Autodesk Inventor part; units mm, degrees
ref_plane "YZ Plane" through (0, 0, 0) normal (1, 0, 0) x (0, 1, 0)
ref_plane "XZ Plane" through (0, 0, 0) normal (0, 1, 0) x (-1, 0, 0)
ref_plane "XY Plane" through (0, 0, 0) normal (0, 0, 1) x (1, 0, 0)
sketch "Sketch2" plane through (0, 0, 0) normal (0, 0, 1) x (1, 0, 0)
  circle A0 centre (0, 0) radius 18.5
  circle A1 centre (38, 0) radius 6.3
  circle A2 centre (0, 0) radius 6.3
  circle A3 centre (38, 0) radius 18.5
  line L0 (-1.1534, 0) -> (34.5511, 0)
  arc A4 (12.005, 14.0759) -> (25.995, 14.0759) centre (19, 22.2775) ccw
  arc A5 (25.995, -14.0759) -> (12.005, -14.0759) centre (19, -22.2775) ccw
  line L1 (1.1428, -18.5) -> (0, -18.5)
  line L2 (1.1428, 18.5) -> (0, 18.5)
  point P0 (38, 18.5)
  point P1 (38, -18.5)
  point P2 (18.5, 0)
  dimension "d0" = 37
  dimension "d19" = 12.6
  dimension "d20" = 37
  dimension "d26" = 38
extrude "Extrusion1" add sketch "Sketch2" along normal blind 4.3
sketch "Sketch3" plane through (0, 0, 4.3) normal (0, 0, 1) x (1, 0, 0)
  circle A0 centre (38, 0) radius 6.3
  line L0 (38, 0) -> (38, 2.8384)
  point P0 (0, 0)
  point P1 (46.7, 0)
  point P2 (18.9, 0)
  dimension "d7" = 27.8
  dimension "d16" = 8.7
hole "Hole1" at (46.7, 0, 4.3) at (18.9, 0, 4.3) direction (0, 0, -1) diameter 2 depth 7
sketch "Sketch4" plane through (0, 0, 0) normal (0, 0, -1) x (-1, 0, 0)
  circle A0 centre (0, 0) radius 6.3
  line L0 (0, 3.334) -> (0, -2.474)
  line L1 (-2.132, 0) -> (2.0257, 0)
  line L2 (-4.2951, 19.0635) -> (4.2951, 19.0635)
  line L3 (4.2951, 19.0635) -> (4.2951, -19.0635)
  line L4 (4.2951, -19.0635) -> (-4.2951, -19.0635)
  line L5 (-4.2951, -19.0635) -> (-4.2951, 19.0635)
  point P0 (4.2951, -4.609)
  point P1 (-4.2951, -4.609)
  point P2 (-4.2951, 4.609)
  point P3 (4.2951, 4.609)
extrude "Extrusion2" cut sketch "Sketch4" against normal blind 2 contours A0 L5 L2 L3 | L3 L4 L5 A0
sketch "Sketch5" plane through (0, 0, 4.3) normal (0, 0, 1) x (1, 0, 0)
  circle A0 centre (38, 0) radius 6.3
  line L0 (38, 0) -> (38, 11.0593)
  line L1 (38, 0) -> (42.2148, 0)
  line L2 (21.1, 6.5) -> (44.1, 6.5)
  line L3 (44.1, 6.5) -> (44.1, -6.5)
  line L4 (44.1, -6.5) -> (21.1, -6.5)
  line L5 (21.1, -6.5) -> (21.1, 6.5)
  circle A1 centre (46.7, 0) radius 1
  point P0 (0, 0)
  point P1 (44.1, -1.5748)
  point P2 (44.1, 1.5748)
  dimension "d21" = 13
  dimension "d22" = 23
  dimension "d23" = 2.6
extrude "Extrusion3" cut sketch "Sketch5" against normal blind 4.3 contours A0 L0 L2 L3 | L3 L4 L5 L2 L0 A0
fillet "Fillet1" radius 1 14 edges at (19, 11.498, 0) (8.3822, 16.4921, 0) (19, -11.498, 0) (8.3822, -16.4921, 0) (56.5, 0, 0) (-18.5, 0, 0) (19, -11.498, 4.3) (56.5, 0, 4.3) (19, 11.498, 4.3) (-18.5, 0, 4.3) (4.2951, 11.3017, 0) (4.2951, -11.3017, 0) (-4.2951, 11.3017, 0) (-4.2951, -11.3017, 0)
sketch "Sketch7" plane through (0, 0, 2) normal (0, 0, -1) x (-1, 0, 0)
  circle A0 centre (0, 0) radius 6.3
  line L0 (0, 0) -> (0, 23.1769)
  line L1 (0, 0) -> (3.1147, 0)
  point P0 (0, 13.1)
  point P1 (0, -13.1)
  dimension "d28" = 26.2
hole "Hole2" at (0, 13.1, 2) at (0, -13.1, 2) direction (0, 0, 1) diameter 2 depth 2.3
properties part number "firsarm" material "Polystyrene"
Design review of the part built by this model. Coordinates are the model's own, in mm. A direction names the side the tool comes from. Give positions to 0.01 mm unless a question says otherwise; leave off trailing zeros. Order: outer loops, then holes, each group sorted by start corner. A loop starts at its lowest first (then second) coordinate and runs counter-clockwise, first axis right, second up. Notation, with made-up numbers: (13.5, 84.5) - (17.5, 84.5) arc R27 cw to (17.5, 104.5) - close; hole circle Ø11 at (-35, 73). An arc over 180 degrees is marked (long way). Write item = value, one per line. Start each with the question number.
Q1. Tool access review of faces 5 (the face through (18.9, -11.5, 2.1)), 6 (the face through (0.1, 11.7, 2)), 7 (the face through (33, -6.5, 2)): name each direction out of +Z, -Z, +X, -X, +Y, -Y from which nothing blocks a thin tool from reaching the whole face with its end or side.
Q2. Clearance check with flat-ended pins moving along their axes: pin 1 Ø1.5 at (y, z) = (-7.5, 2.5) entering from +X; pin 2 Ø1.6 at (x, y) = (18.9, 0) entering from -Z; pin 3 Ø1 at (y, z) = (-11.5, 1) entering from -X; pin 4 Ø2 at (y, z) = (3, 3) entering from -X. State where each tip first meets the part, or that it passes through.
Q3. To check wall thickness, follow L1, parallel to Y at x = 0, z = 2.9; L2, parallel to Y at x = 18.9, z = 1.05; L3, parallel to X at y = -0.5, z = 1.65. State the ranges of each line that lie inside material, in increasing order. Write a range as from..to.
Q4. We need section B-B on y = 0. State the section outline as (x, z) points, plus the area to 3 significant figures.
Q5. We need section A-A on x = 38. State the section outline as (y, z) points.
Q6. Mouldability with a two-part tool opening along Y and no side actions: class faces 1 (the face through (0, -11, 2)), 2 (the face through (-6.294, -0.277, 2.598)), 3 (the face through (47.676, 0.217, 2.12)), 4 (the face through (19.1, 11.5, 2.1)) as released by +Y, released by -Y, zero draft, split by the parting line, or undercut.
Working result:
q1.face_5 = +Z, -Z, -Y
q1.face_6 = -Z, +Y, -Y
q1.face_7 = +Z, -Z
q2.pin_1 = 55.22
q2.pin_2 = through
q2.pin_3 = -14.87
q2.pin_4 = -18.39
q3.L1 = -18.5..-14.1, -12.1..-6.3, 6.3..12.1, 14.1..18.5
q3.L2 = -11.5..-1, 1..11.5
q3.L3 = -18.49..-6.28, 6.28..18.03, 19.77..21.1, 44.28..45.83, 47.57..56.49
q4.outline = (-18.5, 1) arc R1 ccw to (-17.5, 0) - (-6.3, 0) - (-6.3, 4.3) - (-17.5, 4.3) arc R1 ccw to (-18.5, 3.3) - close; (6.3, 0) - (17.9, 0) - (17.9, 4.3) - (6.3, 4.3) - close; (19.9, 0) - (21.1, 0) - (21.1, 4.3) - (19.9, 4.3) - close; (44.3, 0) - (45.7, 0) - (45.7, 4.3) - (44.3, 4.3) - close; (47.7, 0) - (55.5, 0) arc R1 ccw to (56.5, 1) - (56.5, 3.3) arc R1 ccw to (55.5, 4.3) - (47.7, 4.3) - close
q4.area = 151 mm²
q5.outline = (-18.5, 1) arc R1 ccw to (-17.5, 0) - (-6.5, 0) - (-6.5, 4.3) - (-17.5, 4.3) arc R1 ccw to (-18.5, 3.3) - close; (6.5, 0) - (17.5, 0) arc R1 ccw to (18.5, 1) - (18.5, 3.3) arc R1 ccw to (17.5, 4.3) - (6.5, 4.3) - close
q6.face_1 = zero draft
q6.face_2 = undercut
q6.face_3 = undercut
q6.face_4 = released by +Y
